```python
from build123d import *

# Parameters (mm, degrees)
BOSS_EXTRUDE1_DEPTH = 11.5
BOSS_EXTRUDE2_DEPTH = 3.5
SKETCH4_R           = 1.5
BOSS_EXTRUDE3_DEPTH = 3
SKETCH5_R           = 1.25
CUT_EXTRUDE1_DEPTH  = 3.5
SKETCH6_W           = 4
SKETCH6_H           = 11.5
CUT_EXTRUDE2_DEPTH  = 10
SKETCH7_W           = 4
SKETCH7_H           = 11.5
CUT_EXTRUDE3_DEPTH  = 10


with BuildPart() as part:
    # Sketch1 → Boss-Extrude1 (new body)
    with BuildSketch(Plane(origin=(0, 0, 0), x_dir=(1, 0, 0), z_dir=(0, 1, 0))):
        Polygon((-20, 0), (-24, 0), (-24, 22), (-20, 22), (-20, 26), (-18, 26), (-18, 22), (0, 22), (0, 0), (-18, 0), (-18, -4), (-20, -4), align=None)
    extrude(amount=BOSS_EXTRUDE1_DEPTH)

    # Sketch2 → Boss-Extrude2 (add)
    with BuildSketch(Plane.ZY.offset(24)):
        with BuildLine():
            ThreePointArc((-11.140964663, 3.75), (0, 5.75), (-11.140964663, 7.75))
            ThreePointArc((-11.140964663, 7.75), (-13.140964663, 5.75), (-11.140964663, 3.75))
        make_face()
    extrude(amount=BOSS_EXTRUDE2_DEPTH)

    # Sketch4 → Boss-Extrude3 (add)
    with BuildSketch(Plane.ZY.offset(27.5)):
        with Locations((-5.75, 5.75)):
            Circle(SKETCH4_R)
    extrude(amount=BOSS_EXTRUDE3_DEPTH)

    # Sketch5 → Cut-Extrude1 (cut)
    with BuildSketch(Plane.ZY.offset(20)):
        with Locations((-24.8, 5.75)):
            Circle(SKETCH5_R)
        with Locations((2.8, 5.75)):
            Circle(SKETCH5_R)
    extrude(amount=-CUT_EXTRUDE1_DEPTH, mode=Mode.SUBTRACT)

    # Sketch6 → Cut-Extrude2 (cut)
    with BuildSketch(Plane(origin=(-18, 0, 0), x_dir=(0, 0, -1), z_dir=(1, 0, 0))):
        with Locations((24, 5.75)):
            Rectangle(SKETCH6_W, SKETCH6_H)
    extrude(amount=-CUT_EXTRUDE2_DEPTH, mode=Mode.SUBTRACT)

    # Sketch7 → Cut-Extrude3 (cut)
    with BuildSketch(Plane(origin=(-18, 0, 0), x_dir=(0, 0, -1), z_dir=(1, 0, 0))):
        with Locations((-2, 5.75)):
            Rectangle(SKETCH7_W, SKETCH7_H)
    extrude(amount=-CUT_EXTRUDE3_DEPTH, mode=Mode.SUBTRACT)


solid = part.part
```
Could you check a few things on this model? Use its own coordinates, in mm. A direction names the side the tool comes from. Coordinates: 2 decimals unless noted, no trailing zeros. Loops run counter-clockwise (first coordinate to the right, second up) from the corner with the lowest first, then second, coordinate; pieces in that order, holes last.
1) Imagine slicing it at B-B (z = -16.5). List the corners of the cut face in (x, y) for me.
Reported:
outline: (-24, 0) - (0, 0) - (0, 11.5) - (-24, 11.5) - close
2) Please list where these lines run through material, in increasing order: line 1 along X through (y, z) = (10.75, -19.5); line 2 along X through (y, z) = (4.5, -12.5); line 3 along Y through (x, z) = (-27, -7.75).
Reported:
line 1: x = -24 to 0
line 2: x = -27.5 to 0
line 3: y = 0.36 to 11.14
3) Will this pin go through, and if not, where does the flat tip stop? pin 1 Ø1.7 at (y, z) = (3.5, -3.5) entering from -X.
Reported:
pin 1: stops at x = -27.5
4) Imagine slicing it at D-D (y = 6.75). List the corners of the cut face in (x, z) for me, and give its area (3 significant figures).
Reported:
outline: (-30.5, -6.87) - (-27.5, -6.87) - (-27.5, -12.87) - (-24, -12.87) - (-24, -22) - (0, -22) - (0, 0) - (-24, 0) - (-24, -0.09) - (-27.5, -0.09) - (-27.5, -4.63) - (-30.5, -4.63) - close
area: 579 mm2
5) Imagine slicing it at A-A (y = 9). List the corners of the cut face in (x, z) for me.
Reported:
outline: (-27.5, -10.49) - (-24, -10.49) - (-24, -22) - (0, -22) - (0, 0) - (-24, 0) - (-24, -1.01) - (-27.5, -1.01) - close
6) Imagine slicing it at C-C (x = -27). List the corners of the cut face in (y, z) for me, and give its area (3 significant figures).
Reported:
outline: (3.75, -11.14) arc R2 ccw to (7.75, -11.14) arc R5.75 ccw (long way) to start
area: 109 mm2
7) Which directions (+Z, -Z, +X, -X, +Y, -Y) give clear straight access to the entire face, cutting with the end or side of a thin tool? Please do faces 1 (the face through (-24, 10, -1)), 2 (the face through (-27.5, 7, -7)), 3 (the face through (-24, 1, -1)).
Reported:
face 1: +Z, -X, +Y
face 2: -X
face 3: +Z, -X, -Y
